from build123d import *

# Parameters (mm, degrees)
SKETCH1_W           = 220
SKETCH1_H           = 53
SKETCH1_R           = 1.505
SKETCH1_R_2         = 6.315
SKETCH1_R_3         = 3.078429052
SKETCH1_R_4         = 2.929841002
SKETCH1_R_5         = 2.275
SKETCH1_R_6         = 5
BOSS_EXTRUDE1_DEPTH = 5


with BuildPart() as part:
    # Sketch1 → Boss-Extrude1 (new body)
    with BuildSketch(Plane(origin=(0, 0, 0), x_dir=(1, 0, 0), z_dir=(0, 1, 0))):
        with Locations((-42.86437247, 16.587044534)):
            Rectangle(SKETCH1_W, SKETCH1_H)
        with Locations((56.13562753, 38.907044534)):
            Circle(SKETCH1_R, mode=Mode.SUBTRACT)
        with Locations((52.12562753, 38.907044534)):
            Circle(SKETCH1_R, mode=Mode.SUBTRACT)
        with Locations((48.11562753, 38.907044534)):
            Circle(SKETCH1_R, mode=Mode.SUBTRACT)
        with Locations((-141.87437247, 38.907044534)):
            Circle(SKETCH1_R, mode=Mode.SUBTRACT)
        with Locations((-137.87437247, 38.907044534)):
            Circle(SKETCH1_R, mode=Mode.SUBTRACT)
        with Locations((-133.87437247, 38.907044534)):
            Circle(SKETCH1_R, mode=Mode.SUBTRACT)
        with Locations((-42.86437247, 28.997993636)):
            Circle(SKETCH1_R_2, mode=Mode.SUBTRACT)
        with Locations((-42.86437247, 3.997993636)):
            Circle(SKETCH1_R_2, mode=Mode.SUBTRACT)
        with Locations((47.6973107, 10.127310686)):
            Circle(SKETCH1_R_3, mode=Mode.SUBTRACT)
        with Locations((47.6973107, -5.372689314)):
            Circle(SKETCH1_R_4, mode=Mode.SUBTRACT)
        with Locations((36.4973107, 3.997993636)):
            Circle(SKETCH1_R_5, mode=Mode.SUBTRACT)
        with Locations((26.4973107, 3.997993636)):
            Circle(SKETCH1_R_6, mode=Mode.SUBTRACT)
        with Locations((-133.426055639, -5.372689314)):
            Circle(SKETCH1_R_4, mode=Mode.SUBTRACT)
        with Locations((-133.426055639, 10.127310686)):
            Circle(SKETCH1_R_3, mode=Mode.SUBTRACT)
        with Locations((-122.226055639, 3.997993636)):
            Circle(SKETCH1_R_5, mode=Mode.SUBTRACT)
        with Locations((-112.226055639, 3.997993636)):
            Circle(SKETCH1_R_6, mode=Mode.SUBTRACT)
        with BuildLine():
            Line((-52.39437247, 23.161197849), (-52.39437247, 11.591197849))
            ThreePointArc((-52.39437247, 11.591197849), (-50.63437247, 9.831197849), (-48.87437247, 11.591197849))
            Line((-48.87437247, 11.591197849), (-48.87437247, 23.161197849))
            ThreePointArc((-48.87437247, 23.161197849), (-50.63437247, 24.921197849), (-52.39437247, 23.161197849))
        make_face(mode=Mode.SUBTRACT)
        with BuildLine():
            Line((-36.85437247, 23.161197849), (-36.85437247, 11.591197849))
            ThreePointArc((-36.85437247, 11.591197849), (-35.09437247, 9.831197849), (-33.33437247, 11.591197849))
            Line((-33.33437247, 11.591197849), (-33.33437247, 23.161197849))
            ThreePointArc((-33.33437247, 23.161197849), (-35.09437247, 24.921197849), (-36.85437247, 23.161197849))
        make_face(mode=Mode.SUBTRACT)
    extrude(amount=BOSS_EXTRUDE1_DEPTH)


solid = part.part
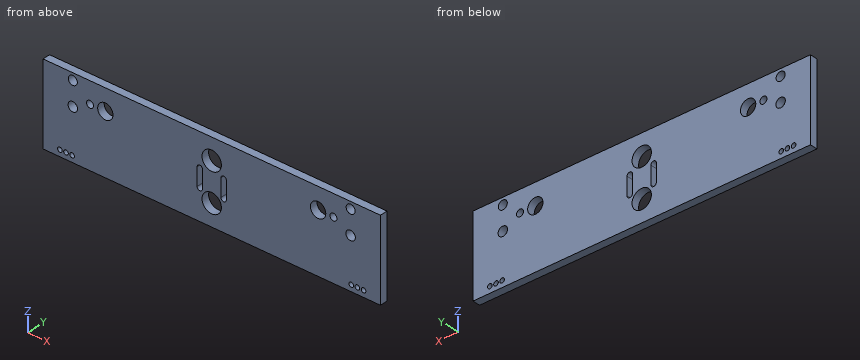
Geometry: final body of the model. Coordinates: model frame, mm. Round coordinates to 2 decimals unless told otherwise and drop trailing zeros. Loops run counter-clockwise (first coordinate to the right, second up) from the corner with the lowest first, then second, coordinate; pieces in that order, holes last. Notation, with made-up numbers: M 3.5,79.5 L 20.5,79.5 A9 ccw 20.5,84.5 Z; hole C 71,2.5 d4. An arc over 180 degrees is marked long. Put each result on its own line as item: value. Start each with the question number.
(1) Section query D-D (x = 26). Return loops of the section in (y, z), then the cut area to 3 significant figures.
(2) Section query A-A (z = -17). Return loops of the section in (x, y).
(3) Section query C-C (y = 0.95). State how many separate pieces and enclosed holes the cut face has, then the cut area to 3 significant figures.
(4) Section query B-B (x = -110). Return loops of the section in (y, z).
(5) Material intervals for line 1 along X through (y, z) = (2.35, -4); line 2 along X through (y, z) = (4, 5.5); line 3 along Z through (x, y) = (27, 3.6), sorted ascending. Write a range as [from, to].
Findings below:
1. outline: M 0,-43.09 L 5,-43.09 L 5,-8.97 L 0,-8.97 Z; M 0,0.98 L 5,0.98 L 5,9.91 L 0,9.91 Z
1. area: 215 mm2
2. outline: M -152.86,0 L -52.39,0 L -52.39,5 L -152.86,5 Z; M -48.87,0 L -36.85,0 L -36.85,5 L -48.87,5 Z; M -33.33,0 L 67.14,0 L 67.14,5 L -33.33,5 Z
3. separate pieces: 1
3. enclosed holes: 18
3. area: 11,000 mm2
4. outline: M 0,-43.09 L 5,-43.09 L 5,-8.48 L 0,-8.48 Z; M 0,0.48 L 5,0.48 L 5,9.91 L 0,9.91 Z
5. line 1: x = [-152.86, -124.5], [-119.95, -117.23], [-107.23, -49.18], [-36.55, 21.5], [31.5, 34.22], [38.77, 67.14]
5. line 2: x = [-152.86, -136.35], [-130.5, 44.77], [50.62, 67.14]
5. line 3: z = [-43.09, -8.97], [0.98, 9.91]
